Can you work these out from the model? Positions are in its coordinate system, mm. Give positions to 0.01 mm unless a question says otherwise; leave off trailing zeros. Loops run counter-clockwise (first coordinate to the right, second up) from the corner with the lowest first, then second, coordinate; pieces in that order, holes last. Notation, with made-up numbers: (42.25, 45) -> (55.25, 45) arc R28 cw to (55.25, 81) -> close; hole circle Ø10 at (9, 17). An arc over 180 degrees is marked (long way). Return JSON: item names as keys, results as strings. Group by question number.
Q1. Suppose I cut it at C-C, the plane z = 1.9. Count the separate pieces of the cut face and the enclosed holes in it, and give its area (3 significant figures).
Q2. Suppose I cut it at B-B, the plane y = 4.5. Please give me the cut outline in (x, z), and give its area (3 significant figures).
Q3. Suppose I cut it at A-A, the plane x = -26.2. Please give me the cut outline in (y, z), and give its area (3 significant figures).
Q4. I need wall thicknesses on line 1 along Y through (x, z) = (91.4, 1.85); line 2 along X through (y, z) = (6, 1.25); line 3 along Y through (x, z) = (-11.5, 0.4). Which ranges of each line are inside material? Lowest first, please. Write a range as [from, to].
Autodesk Inventor part; units mm, degrees
ref_plane "YZ Plane" through (0, 0, 0) normal (1, 0, 0) x (0, 1, 0)
ref_plane "XZ Plane" through (0, 0, 0) normal (0, 1, 0) x (-1, 0, 0)
ref_plane "XY Plane" through (0, 0, 0) normal (0, 0, 1) x (1, 0, 0)
sketch "Sketch1" plane through (0, 0, 0) normal (0, 0, 1) x (1, 0, 0)
  line L0 (-30, -15) -> (-30, 15)
  line L1 (-30, 15) -> (120, 15)
  line L2 (120, 15) -> (120, -15)
  line L3 (120, -15) -> (-30, -15)
  line L4 (-60, 0) -> (150, 0)
  line L5 (0, -21) -> (0, 21)
  dimension "d13" = 30
  dimension "d55" = 150
  dimension "d56" = 15
extrude "Extrusion1" add sketch "Sketch1" along normal blind 2.8
sketch "Sketch4" plane through (0, 0, 2.8) normal (0, 0, 1) x (1, 0, 0)
  line L0 (-60, 0) -> (150, 0)
  line L1 (17.9, 9.9) -> (17.9, 2.5)
  line L2 (-22.4, 9.9) -> (17.9, 9.9)
  line L3 (17.9, 2.5) -> (23.9, 2.5)
  line L4 (23.9, 2.5) -> (23.9, -2.5)
  line L5 (23.9, -2.5) -> (17.9, -2.5)
  line L6 (17.9, -2.5) -> (17.9, -9.9)
  line L7 (17.9, -9.9) -> (-22.4, -9.9)
  line L8 (-22.4, -9.9) -> (-22.4, 9.9)
  line L9 (-22.4, 9.9) -> (17.9, 9.9)
  circle A0 centre (26.7, 0) radius 1.5
  circle A1 centre (-26.2, 0) radius 1.5
  line L10 (120, 15) -> (120, -15)
  line L11 (120, -15) -> (-30, -15)
  line L12 (112.8, 2.5) -> (115, 2.5)
  line L13 (115, 2.5) -> (115, -2.5)
  line L14 (115, -2.5) -> (112.8, -2.5)
  line L15 (112.8, -2.5) -> (112.8, 2.5)
  line L16 (97.8, 2.5) -> (100, 2.5)
  line L17 (100, 2.5) -> (100, -2.5)
  line L18 (100, -2.5) -> (97.8, -2.5)
  line L19 (97.8, -2.5) -> (97.8, 2.5)
  line L20 (82.8, 2.5) -> (85, 2.5)
  line L21 (85, 2.5) -> (85, -2.5)
  line L22 (85, -2.5) -> (82.8, -2.5)
  line L23 (82.8, -2.5) -> (82.8, 2.5)
  line L24 (67.8, 2.5) -> (70, 2.5)
  line L25 (70, 2.5) -> (70, -2.5)
  line L26 (70, -2.5) -> (67.8, -2.5)
  line L27 (67.8, -2.5) -> (67.8, 2.5)
  line L28 (52.8, 2.5) -> (55, 2.5)
  line L29 (55, 2.5) -> (55, -2.5)
  line L30 (55, -2.5) -> (52.8, -2.5)
  line L31 (52.8, -2.5) -> (52.8, 2.5)
  line L32 (37.8, 2.5) -> (40, 2.5)
  line L33 (40, 2.5) -> (40, -2.5)
  line L34 (40, -2.5) -> (37.8, -2.5)
  line L35 (37.8, -2.5) -> (37.8, 2.5)
  line L36 (112.8, -7.5) -> (115, -7.5)
  line L37 (115, -7.5) -> (115, -12.5)
  line L38 (115, -12.5) -> (112.8, -12.5)
  line L39 (112.8, -12.5) -> (112.8, -7.5)
  line L40 (97.8, -7.5) -> (100, -7.5)
  line L41 (100, -7.5) -> (100, -12.5)
  line L42 (100, -12.5) -> (97.8, -12.5)
  line L43 (97.8, -12.5) -> (97.8, -7.5)
  line L44 (82.8, -7.5) -> (85, -7.5)
  line L45 (85, -7.5) -> (85, -12.5)
  line L46 (85, -12.5) -> (82.8, -12.5)
  line L47 (82.8, -12.5) -> (82.8, -7.5)
  line L48 (67.8, -7.5) -> (70, -7.5)
  line L49 (70, -7.5) -> (70, -12.5)
  line L50 (70, -12.5) -> (67.8, -12.5)
  line L51 (67.8, -12.5) -> (67.8, -7.5)
  line L52 (52.8, -7.5) -> (55, -7.5)
  line L53 (55, -7.5) -> (55, -12.5)
  line L54 (55, -12.5) -> (52.8, -12.5)
  line L55 (52.8, -12.5) -> (52.8, -7.5)
  line L56 (37.8, -7.5) -> (40, -7.5)
  line L57 (40, -7.5) -> (40, -12.5)
  line L58 (40, -12.5) -> (37.8, -12.5)
  line L59 (37.8, -12.5) -> (37.8, -7.5)
  line L60 (112.8, 12.5) -> (112.8, 7.5)
  line L61 (115, 12.5) -> (112.8, 12.5)
  line L62 (112.8, 7.5) -> (115, 7.5)
  line L63 (115, 7.5) -> (115, 12.5)
  line L64 (97.8, 12.5) -> (97.8, 7.5)
  line L65 (100, 12.5) -> (97.8, 12.5)
  line L66 (97.8, 7.5) -> (100, 7.5)
  line L67 (100, 7.5) -> (100, 12.5)
  line L68 (82.8, 12.5) -> (82.8, 7.5)
  line L69 (85, 12.5) -> (82.8, 12.5)
  line L70 (82.8, 7.5) -> (85, 7.5)
  line L71 (85, 7.5) -> (85, 12.5)
  line L72 (67.8, 12.5) -> (67.8, 7.5)
  line L73 (70, 12.5) -> (67.8, 12.5)
  line L74 (67.8, 7.5) -> (70, 7.5)
  line L75 (70, 7.5) -> (70, 12.5)
  line L76 (52.8, 12.5) -> (52.8, 7.5)
  line L77 (55, 12.5) -> (52.8, 12.5)
  line L78 (52.8, 7.5) -> (55, 7.5)
  line L79 (55, 7.5) -> (55, 12.5)
  line L80 (37.8, 12.5) -> (37.8, 7.5)
  line L81 (40, 12.5) -> (37.8, 12.5)
  line L82 (37.8, 7.5) -> (40, 7.5)
  line L83 (40, 7.5) -> (40, 12.5)
  circle A2 centre (106.4, 0) radius 1.5
  circle A3 centre (91.4, 0) radius 1.5
  circle A4 centre (76.4, 0) radius 1.5
  circle A5 centre (61.4, 0) radius 1.5
  circle A6 centre (46.4, 0) radius 1.5
  dimension "d57" = 2.2
  dimension "d58" = 5
  dimension "d59" = 2.5
  dimension "d60" = 5
  dimension "d63" = 15
  dimension "d66" = 10
  dimension "d69" = 3
  dimension "d70" = 6.4
  dimension "d73" = 15
extrude "Extrusion3" cut sketch "Sketch4" against normal through all
equation "\"d56\" = 0.5 * d13"
properties part number "Acrylic_UpperArm_Support"
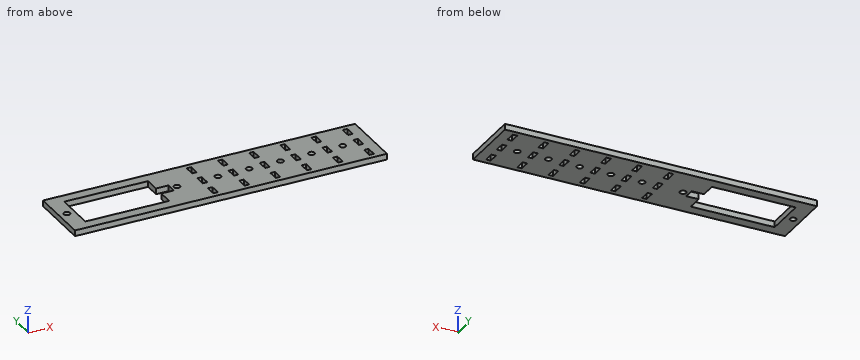
Ans:
{
 "1": {"separate pieces": "1", "enclosed holes": "26", "area": "3,420 mm^2"},
 "2": {"outline": "(-30, 0) -> (-22.4, 0) -> (-22.4, 2.8) -> (-30, 2.8) -> close; (17.9, 0) -> (120, 0) -> (120, 2.8) -> (17.9, 2.8) -> close", "area": "307 mm^2"},
 "3": {"outline": "(-15, 0) -> (-1.5, 0) -> (-1.5, 2.8) -> (-15, 2.8) -> close; (1.5, 0) -> (15, 0) -> (15, 2.8) -> (1.5, 2.8) -> close", "area": "75.6 mm^2"},
 "4": {"line 1": "y = [-15, -1.5], [1.5, 15]", "line 2": "x = [-30, -22.4], [17.9, 120]", "line 3": "y = [-15, -9.9], [9.9, 15]"}
}
